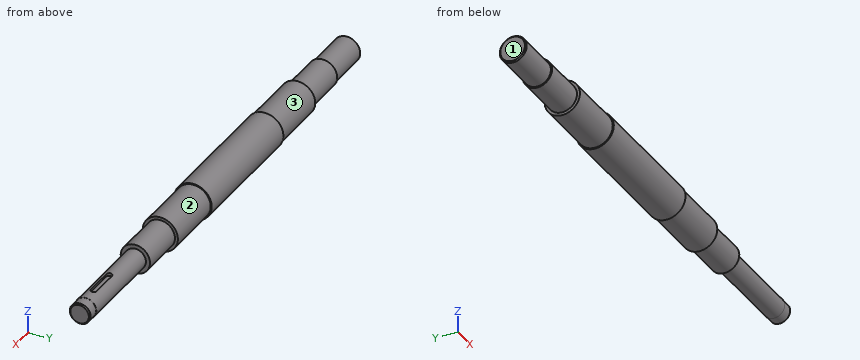
```python
from build123d import *

# Parameters (mm, degrees)
CUT_EXTRUDE_START   = 9
CUT_EXTRUDE_1_DEPTH = 2.5


with BuildPart() as part:
    # 草圖1 → 旋轉1 (revolve)
    with BuildSketch(Plane.XY, mode=Mode.PRIVATE) as revolve_1_sk:
        Polygon((57.8, 15.875), (-57.8, 15.875), (-57.8, 15), (-110.8, 15), (-110.8, 12.5), (-151, 12.5), (-151, 11.5), (-190, 11.5), (-191, 10.5), (-191, 0), (241, 0), (241, 7.9), (240, 8.9), (231, 8.9), (231, 9), (151, 9), (151, 12.5), (110.8, 12.5), (110.8, 15), (57.8, 15), align=None)
    revolve(revolve_1_sk.sketch.rotate(Axis((0, 0, 0), (1, 0, 0)), 90), axis=Axis((0, 0, 0), (1, 0, 0)))

    # 草圖2 → 除料-伸長1 (cut)
    with BuildSketch(Plane.XY.offset(CUT_EXTRUDE_START)):
        with BuildLine():
            Line((193.5, 2.5), (218.5, 2.5))
            ThreePointArc((218.5, 2.5), (221, 0), (218.5, -2.5))
            Line((218.5, -2.5), (193.5, -2.5))
            ThreePointArc((193.5, -2.5), (191, 0), (193.5, 2.5))
        make_face()
    extrude(amount=-CUT_EXTRUDE_1_DEPTH, mode=Mode.SUBTRACT)


solid = part.part
```
Input: part model. Units: mm. Frame: model coordinates. Face numbers are marked on the shaded views. A direction names the side the tool comes from. Round coordinates to 2 decimals unless told otherwise and drop trailing zeros. Loops run counter-clockwise (first coordinate to the right, second up) from the corner with the lowest first, then second, coordinate; pieces in that order, holes last.
1) Pin query (flat end, axial travel): pin 1 (8 mm diameter, centred on x = -107.5, y = 8, fed in from +Z); pin 2 (4 mm diameter, centred on x = 161.5, y = -0.5, fed in from -Z); pin 3 (8 mm diameter, centred on x = -3.5, y = -3, fed in from -Z) (3 decimals); pin 4 (4 mm diameter, centred on x = 9, y = 2.5, fed in from +Z). Return the tip coordinate at first contact, or that it passes through.
Ans:
pin 1: stops at z = 14.46
pin 2: stops at z = -9
pin 3: stops at z = -15.875
pin 4: stops at z = 15.87
2) Section query B-B on x = 64. Return the cut outline in (y, z).
Ans:
outline: circle Ø30 at (0, 0)
3) Material intervals for line 1 (X direction, y = 1, z = 13.5); line 2 (X direction, y = 6, z = 10.5); line 3 (Y direction, x = -87.5, z = 0.5), sorted ascending.
Ans:
line 1: x = -110.8 to 110.8
line 2: x = -151 to 151
line 3: y = -14.99 to 14.99
4) Section query A-A on x = -4. Return the cut outline in (y, z) (3 decimals), plus the area to 3 significant figures.
Ans:
outline: circle Ø31.75 at (0, 0)
area: 792 mm2
5) Set-up query: the marked faces 1, 2 and 3. Return all of +Z, -Z, +X, -X, +Y, -Y with unobstructed straight access to the full face (end or side cutting, diameter ignored); none if empty.
Ans:
face 1: +Z, -Z, -X, +Y, -Y
face 2: +X
face 3: -X
